```python
from build123d import *

# Parameters (mm, degrees)
SKETCH1_R           = 85
SKETCH1_R_2         = 82
BOSS_EXTRUDE1_DEPTH = 1200
SKETCH2_R           = 1.25
CUT_EXTRUDE1_DEPTH  = 900
CIRPATTERN1_COUNT   = 4
SKETCH3_W           = 6
SKETCH3_H           = 6
SKETCH3_H_2         = 10
CUT_EXTRUDE2_DEPTH  = 104
CIRPATTERN2_COUNT   = 2
SKETCH5_R           = 1
CUT_EXTRUDE3_DEPTH  = 104
CIRPATTERN3_COUNT   = 4


with BuildPart() as part:
    # Sketch1 → Boss-Extrude1 (new body)
    with BuildSketch(Plane.XY):
        Circle(SKETCH1_R)
        Circle(SKETCH1_R_2, mode=Mode.SUBTRACT)
    extrude(amount=BOSS_EXTRUDE1_DEPTH)

    # Sketch2 → Cut-Extrude1 (cut)
    with BuildSketch(Plane(origin=(0, 0, 0), x_dir=(1, 0, 0), z_dir=(0, 1, 0))):
        with Locations(Location((0, -393, 0), (0, 0, 270))):
            Circle(SKETCH2_R)
    cut_extrude1 = extrude(amount=-CUT_EXTRUDE1_DEPTH, mode=Mode.SUBTRACT)

    # CirPattern1: Cut-Extrude1 ×4 about axis
    cirpattern1_axis = Axis((0, 0, 0), (0, 0, 1))
    for i in range(1, CIRPATTERN1_COUNT):
        add(cut_extrude1.rotate(cirpattern1_axis, i * 360 / CIRPATTERN1_COUNT), mode=Mode.SUBTRACT)

    # Sketch3 → Cut-Extrude2 (cut)
    with BuildSketch(Plane(origin=(0, 0, 0), x_dir=(1, 0, 0), z_dir=(0, 1, 0))):
        with Locations((0, -30)):
            Rectangle(SKETCH3_W, SKETCH3_H)
        with Locations((0, -38)):
            Rectangle(SKETCH3_W, SKETCH3_H_2)
    cut_extrude2 = extrude(amount=-CUT_EXTRUDE2_DEPTH, mode=Mode.SUBTRACT)

    # CirPattern2: Cut-Extrude2 ×2 about axis
    cirpattern2_axis = Axis((0, 0, 0), (0, 0, 1))
    for i in range(1, CIRPATTERN2_COUNT):
        add(cut_extrude2.rotate(cirpattern2_axis, i * 360 / CIRPATTERN2_COUNT), mode=Mode.SUBTRACT)

    # Sketch5 → Cut-Extrude3 (cut)
    with BuildSketch(Plane(origin=(0, 0, 0), x_dir=(1, 0, 0), z_dir=(0, 1, 0))):
        with Locations(Location((0, -63.5, 0), (0, 0, 270))):
            Circle(SKETCH5_R)
    cut_extrude3 = extrude(amount=-CUT_EXTRUDE3_DEPTH, mode=Mode.SUBTRACT)

    # CirPattern3: Cut-Extrude3 ×4 about axis
    cirpattern3_axis = Axis((0, 0, 0), (0, 0, 1))
    for i in range(1, CIRPATTERN3_COUNT):
        add(cut_extrude3.rotate(cirpattern3_axis, i * 360 / CIRPATTERN3_COUNT), mode=Mode.SUBTRACT)


solid = part.part
```
Verification items for the finished model (mm, model axes). Round coordinates to 2 decimals unless told otherwise and drop trailing zeros. Order: outer loops, then holes, each group sorted by start corner. A loop starts at its lowest first (then second) coordinate and runs counter-clockwise, first axis right, second up. Notation, with made-up numbers: (15.25, -40) -> (23.25, -40) arc R28 cw to (23.25, -5) -> close; hole circle Ø10 at (-14.75, -20.75). An arc over 180 degrees is marked (long way). Put each result on its own line as item: value. Start each with the question number.
(1) Section check A-A (y = 32.5). Enter the section's corners in (x, z).
(2) Draft check along Y on faces 1 (the face through (-18, -80, 592)), 2 (the face through (-67.453, -51.721, 591.6)), 3 (the face through (-44, 70, 0)). Enter one of: +Y half, -Y half, draft (parallel to the pull), parting line (faces both ways), or undercut.
(3) Section check B-B (z = 887). Enter the section's corners in (x, y), then the cut area to 3 significant figures.
(4) Section check C-C (x = 44). Enter the section's corners in (y, z), then the cut area to 3 significant figures.
(5) Material ranges on line 1 along Z through (x, y) = (0, -83); line 2 along Z through (x, y) = (84, 0); line 3 along X through (y, z) = (-4.5, 995.5), recorded low to high.
(6) Depth check by flat-ended pin: pin 1 Ø2 at (x, z) = (0, 393) entering from +Y; pin 2 Ø12 at (y, z) = (28, 860.5) entering from -X; pin 3 Ø10 at (y, z) = (31.5, 658.5) entering from -X; pin 4 Ø8 at (y, z) = (-63, 452) entering from -X. Enter the tip coordinate at first touch or a pass-through.
Completed:
1. outline: (-78.54, 0) -> (-75.28, 0) -> (-75.28, 1200) -> (-78.54, 1200) -> close; (75.28, 0) -> (78.54, 0) -> (78.54, 1200) -> (75.28, 1200) -> close
2. face 1: undercut
2. face 2: parting line
2. face 3: draft
3. outline: circle Ø170 at (0, 0); hole circle Ø164 at (0, 0)
3. area: 1,570 mm2
4. outline: (-72.73, 0) -> (-69.2, 0) -> (-69.2, 1200) -> (-72.73, 1200) -> close; (69.2, 0) -> (72.73, 0) -> (72.73, 1200) -> (69.2, 1200) -> close
4. area: 8,470 mm2
5. line 1: z = 0 to 27, 43 to 62.5, 64.5 to 391.75, 394.25 to 1200
5. line 2: z = 0 to 62.5, 64.5 to 391.75, 394.25 to 1200
5. line 3: x = -84.88 to -81.88, 81.88 to 84.88
6. pin 1: passes through
6. pin 2: stops at x = -82.1
6. pin 3: stops at x = -80.76
6. pin 4: stops at x = -61.19
